Geometry: see drawing. Coordinates: mm, zero at the bounding-box minimum. Coordinates: 2 decimals unless noted, no trailing zeros. Write each loop counter-clockwise with the first axis right and the second up, starting at its lowest first coordinate (ties: lowest second). Pieces come first, ordered by that corner, then holes.
1) Section query B-B (x = 81.5). Output: boundary loops of the cut face in (y, z) (1 decimal).
2) Draft query along X for the marked faces 1, 2 and 3. Return one class per face: pulls with the +X half, pulls with the -X half, needs draft (parallel to the pull), parting line crosses it, or undercut.
3) Section query C-C (y = 22.5). Output: boundary loops of the cut face in (x, z), then the cut area to 3 significant figures.
4) Line query: L1, parallel to Z at x = 55, y = 15; L2, parallel to X at y = 30.5, z = 33; L3, parallel to X at y = 23, z = 37 (1 decimal). Output: solid intervals per line, ascending.
5) Section query A-A (y = 32). Output: boundary loops of the cut face in (x, z) (1 decimal), then the cut area to 3 significant figures.
6) Pin query (flat end, axial travel): pin 1 Ø1 at (x, z) = (75, 54) entering from +Y; pin 2 Ø3 at (y, z) = (8.5, 40) entering from -X; pin 3 Ø6 at (x, y) = (37.5, 17.5) entering from +Z. Return the tip coordinate at first contact, or that it passes through.
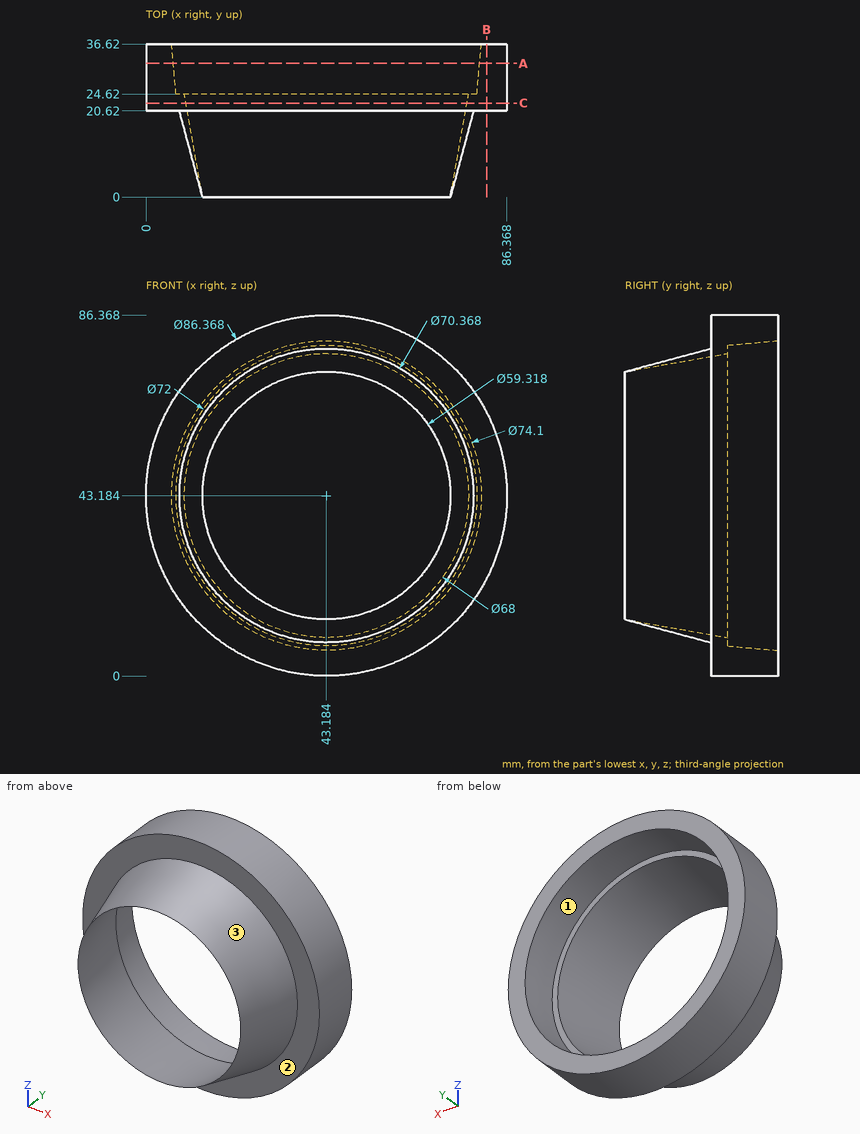
Answer:
1. outline: (20.6, 23.3) - (36.6, 23.3) - (36.6, 63.1) - (20.6, 63.1) - close
2. face 1: undercut
2. face 2: needs draft
2. face 3: parting line crosses it
3. outline: circle Ø86.37 at (43.18, 43.18); hole circle Ø67.25 at (43.18, 43.18)
3. area: 2,310 mm2
4. L1: z = 11.65 to 13.12, 73.25 to 74.72
4. L2: x = 1.22 to 8.12, 78.25 to 85.15
4. L3: x = 0.4 to 10, 76.3 to 85.9
5. outline: circle Ø86.4 at (43.2, 43.2); hole circle Ø73.3 at (43.2, 43.2)
5. area: 1,640 mm2
6. pin 1: stops at y = 24.62
6. pin 2: stops at x = 10.98
6. pin 3: stops at z = 77.98
